Input: dimensioned drawing with shaded views. Units: mm. Origin: part minimum x, y, z. Round coordinates to 2 decimals unless told otherwise and drop trailing zeros. Order: outer loops, then holes, each group sorted by start corner. A loop starts at its lowest first (then second) coordinate and runs counter-clockwise, first axis right, second up. Notation, with made-up numbers: M 26.25,69.25 L 42.25,69.25 A14 ccw 42.25,96.25 Z; hole C 74.5,-13 d8. An arc over 180 degrees is marked long. Put each result on its own line as item: value. Start each with the question number.
1) Section A-A, the plane x = 265. Return loops of the section in (y, z).
2) First-contact query: P1, Ø1.5, axis at y = 91.5, z = 458.5, coming from the -X side. Flat tip, straight axial feed; report the tip coordinate or a pass-through.
3) Section D-D, the plane x = 336.5. Return loops of the section in (y, z), then the cut area to 3 significant figures.
4) Material intervals for probe 1 along Z at (x, y) = (102.5, 82); probe 2 along X at (y, z) = (53.5, 600); probe 3 along X at (y, z) = (55, 914), sorted ascending. Write a range as [from, to].
5) Section C-C, the plane z = 219.5. Return loops of the section in (x, y), then the cut area to 3 significant figures.
6) Section B-B, the plane z = 944. Return loops of the section in (x, y).
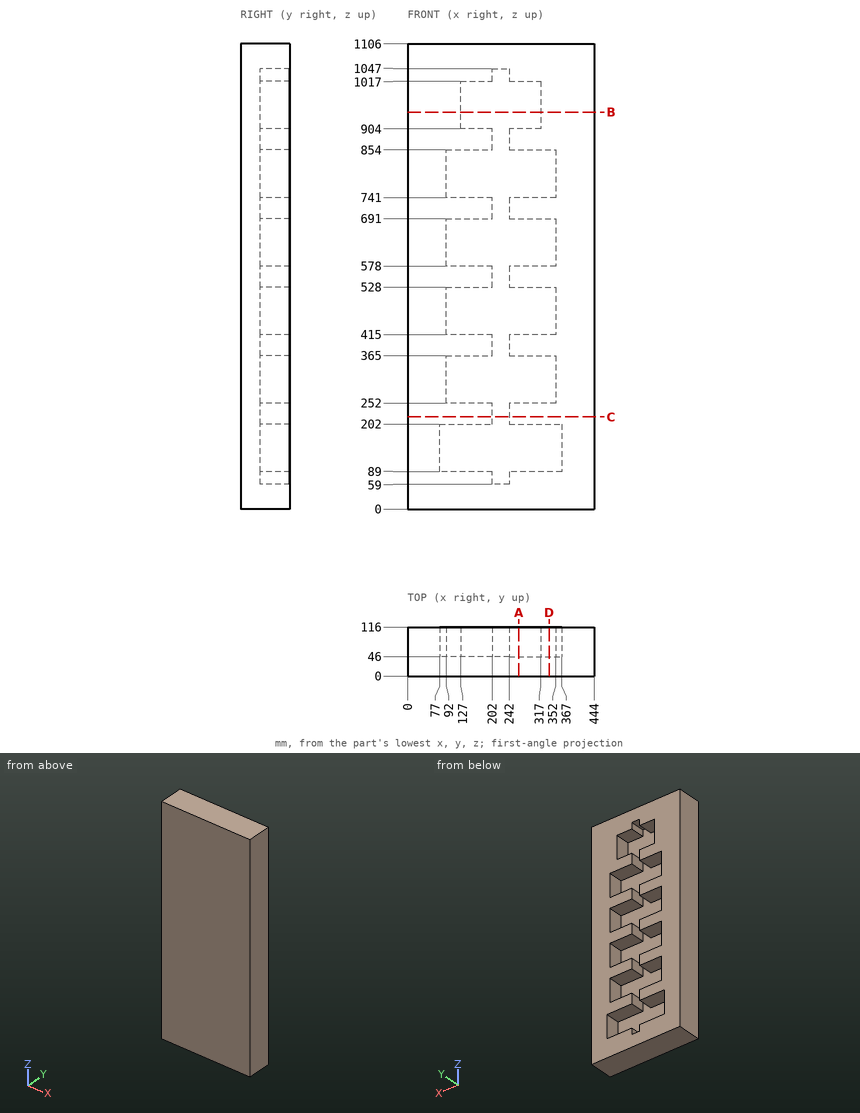
Result sheet:
1. outline: M 0,0 L 116,0 L 116,89 L 46,89 L 46,202 L 116,202 L 116,252 L 46,252 L 46,365 L 116,365 L 116,415 L 46,415 L 46,528 L 116,528 L 116,578 L 46,578 L 46,691 L 116,691 L 116,741 L 46,741 L 46,854 L 116,854 L 116,904 L 46,904 L 46,1017 L 116,1017 L 116,1106 L 0,1106 Z
2. P1: stops at x = 0
3. outline: M 0,0 L 116,0 L 116,89 L 46,89 L 46,202 L 116,202 L 116,252 L 46,252 L 46,365 L 116,365 L 116,415 L 46,415 L 46,528 L 116,528 L 116,578 L 46,578 L 46,691 L 116,691 L 116,741 L 46,741 L 46,854 L 116,854 L 116,1106 L 0,1106 Z
3. area: 88,700 mm2
4. probe 1: z = [0, 89], [202, 252], [365, 415], [528, 578], [691, 741], [854, 1106]
4. probe 2: x = [0, 92], [352, 444]
4. probe 3: x = [0, 127], [317, 444]
5. outline: M 0,0 L 444,0 L 444,116 L 242,116 L 242,46 L 202,46 L 202,116 L 0,116 Z
5. area: 48,700 mm2
6. outline: M 0,0 L 444,0 L 444,116 L 317,116 L 317,46 L 127,46 L 127,116 L 0,116 Z
